Input: part model. Units: mm. Frame: model coordinates. Face numbers are marked on the shaded views. A direction names the side the tool comes from. Give positions to 0.01 mm unless a question says otherwise; leave off trailing zeros. Loops run counter-clockwise (first coordinate to the right, second up) from the corner with the lowest first, then second, coordinate; pieces in that order, holes last. Notation, with made-up numbers: (80.5, 72) - (129.5, 72) arc R16 cw to (129.5, 99) - close; hole circle Ø7 at (23, 78). An arc over 180 degrees is marked (long way). Answer as a JSON object with one key per item and string values. Group by question number.
(1) Material intervals for L1, parallel to Y at x = 4.25, z = 2.25; L2, parallel to X at y = 3, z = 0; L3, parallel to Z at x = 0.25, y = 28.5, sorted ascending.
(2) Access query for the marked faces 1 and 2. Directions: +Z, -Z, +X, -X, +Y, -Y. A direction counts if a zero-diameter tool reaches every point of the face in a straight line with its end or side. Return the directions, or none.
(3) Section query C-C (y = 5). Return loops of the section in (x, z).
(4) Section query B-B (z = 0). Return loops of the section in (x, y), plus the area to 3 significant figures.
(5) Pin query (flat end, axial travel): P1, Ø6, axis at x = -1.5, y = 15.5, coming from the -Z side; P2, Ø4, axis at y = 39, z = -1.5, coming from the -X side; P3, Ø1.5, axis at x = -3, z = 2.5, coming from the -Y side. Return the tip coordinate at first contact, or that it passes through.
(6) Section query A-A (x = 0). Return loops of the section in (y, z).
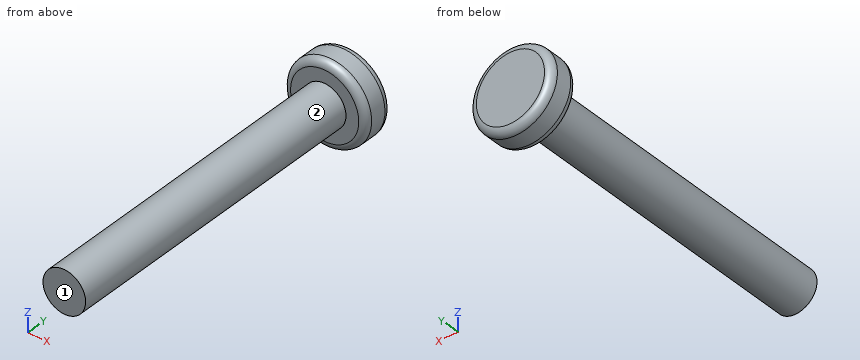
```python
from build123d import *

# Parameters (mm, degrees)
SKETCH1_R           = 3
BOSS_EXTRUDE1_DEPTH = 45
SKETCH2_R           = 5.8
BOSS_EXTRUDE2_DEPTH = 4.3
FILLET1_R           = 1


with BuildPart() as part:
    # Sketch1 → Boss-Extrude1 (new body)
    with BuildSketch(Plane(origin=(0, 0, 0), x_dir=(1, 0, 0), z_dir=(0, 1, 0))):
        with Locations(Location((0, 0, 0), (0, 0, 270))):  # turned: the seam where the file's is
            Circle(SKETCH1_R)
    extrude(amount=BOSS_EXTRUDE1_DEPTH)

    # Sketch2 → Boss-Extrude2 (add)
    with BuildSketch(Plane(origin=(0, 45, 0), x_dir=(1, 0, 0), z_dir=(0, 1, 0))):
        with Locations(Location((0, 0, 0), (0, 0, 270))):  # turned: the seam where the file's is
            Circle(SKETCH2_R)
    extrude(amount=BOSS_EXTRUDE2_DEPTH)

    # Fillet1
    fillet1_edges = [part.edges().sort_by_distance(p)[0] for p in [
        (0, 45, -5.8),
        (0, 49.3, -5.8),
    ]]
    fillet(fillet1_edges, radius=FILLET1_R)


solid = part.part
```
Recorded:
{
 "1": {"L1": "y = 45 to 49.3", "L2": "x = -3 to 3", "L3": "z = -2.99 to 2.99"},
 "2": {"face 1": "+Z, -Z, +X, -X, -Y", "face 2": "-Y"},
 "3": {"outline": "circle Ø6 at (0, 0)"},
 "4": {"outline": "(-5.8, 46) arc R1 ccw to (-4.8, 45) - (-3, 45) - (-3, 0) - (3, 0) - (3, 45) - (4.8, 45) arc R1 ccw to (5.8, 46) - (5.8, 48.3) arc R1 ccw to (4.8, 49.3) - (-4.8, 49.3) arc R1 ccw to (-5.8, 48.3) - close", "area": "319 mm^2"},
 "5": {"P1": "stops at z = -3", "P2": "stops at x = -3", "P3": "stops at y = 45"},
 "6": {"outline": "(0, -3) - (45, -3) - (45, -4.8) arc R1 ccw to (46, -5.8) - (48.3, -5.8) arc R1 ccw to (49.3, -4.8) - (49.3, 4.8) arc R1 ccw to (48.3, 5.8) - (46, 5.8) arc R1 ccw to (45, 4.8) - (45, 3) - (0, 3) - close"}
}
